Check sheet for the modelled part. Datum: model origin and axes. Units: mm. Face numbers are marked on the shaded views. Round coordinates to 2 decimals unless told otherwise and drop trailing zeros. Write each loop counter-clockwise with the first axis right and the second up, starting at its lowest first coordinate (ties: lowest second). Pieces come first, ordered by that corner, then holes. Notation, with made-up numbers: (8, 23) -> (39, 23) arc R20 cw to (39, 37) -> close; hole circle Ø2 at (-28.5, -16.5). An arc over 180 degrees is marked (long way). One line per item, written item: value.
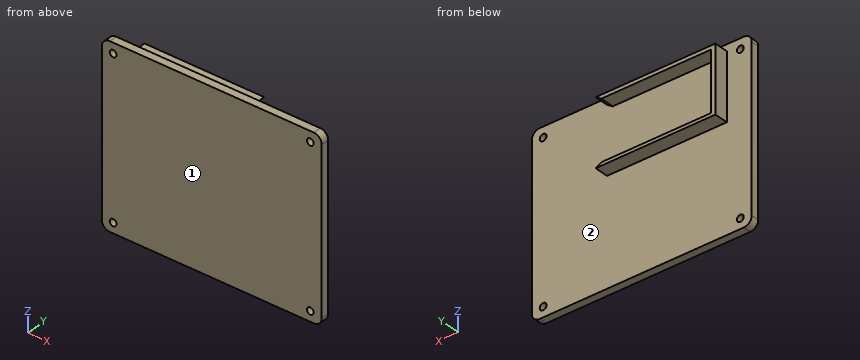
from build123d import *

# Parameters (mm, degrees)
BOSS_EXTRUDE1_DEPTH = 11
SKETCH1_3_R         = 1.7
BOSS_EXTRUDE2_DEPTH = 4


with BuildPart() as part:
    # Sketch1 → Boss-Extrude1 (new body)
    with BuildSketch(Plane(origin=(0, 0, 0), x_dir=(1, 0, 0), z_dir=(0, 1, 0))):
        Polygon((14.535232679, 29.5), (17.346594298, 31.108605337), (-42.592792902, 31.108605337), (-42.592792902, -1.87579117), (17.346594298, -1.87579117), (14.535232679, 0), (-40.464767321, 0), (-40.464767321, 29.5), align=None)
    extrude(amount=BOSS_EXTRUDE1_DEPTH)

    # Sketch1<3> → Boss-Extrude2 (add)
    with BuildSketch(Plane(origin=(0, 0, 0), x_dir=(1, 0, 0), z_dir=(0, 1, 0))):
        with BuildLine():
            Line((55.045, -1.09), (55.045, 79.51))
            ThreePointArc((55.045, 79.51), (53.873427125, 82.338427125), (51.045, 83.51))
            Line((51.045, 83.51), (-51.045, 83.51))
            ThreePointArc((-51.045, 83.51), (-53.873427125, 82.338427125), (-55.045, 79.51))
            Line((-55.045, 79.51), (-55.045, -1.09))
            ThreePointArc((-55.045, -1.09), (-53.873427125, -3.918427125), (-51.045, -5.09))
            Line((-51.045, -5.09), (51.045, -5.09))
            ThreePointArc((51.045, -5.09), (53.873427125, -3.918427125), (55.045, -1.09))
        make_face()
        with Locations((-49.365, 0)):
            Circle(SKETCH1_3_R, mode=Mode.SUBTRACT)
        Polygon((17.346594298, 31.108605337), (14.535232679, 29.5), (-40.464767321, 29.5), (-40.464767321, 0), (14.535232679, 0), (17.346594298, -1.87579117), (-42.592792902, -1.87579117), (-42.592792902, 31.108605337), align=None, mode=Mode.SUBTRACT)
        with Locations((49.365, 0)):
            Circle(SKETCH1_3_R, mode=Mode.SUBTRACT)
        with Locations((-49.365, 78.51)):
            Circle(SKETCH1_3_R, mode=Mode.SUBTRACT)
        with Locations((49.365, 78.51)):
            Circle(SKETCH1_3_R, mode=Mode.SUBTRACT)
    extrude(amount=BOSS_EXTRUDE2_DEPTH)


solid = part.part
Item 1: Sectioned sample at C-C (z = -41). Enter the section's corners in (x, y) (3 decimals).
Result set:
outline: (-55.045, 0) -> (55.045, 0) -> (55.045, 4) -> (-55.045, 4) -> close
Item 2: Depth check by flat-ended pin: pin 1 (5.5 mm diameter, centred on x = -3.5, y = 7, fed in from -Z); pin 2 (3.5 mm diameter, centred on x = -25.5, y = 8.5, fed in from +Z); pin 3 (4 mm diameter, centred on x = -49.365, z = -78.51, fed in from +Y); pin 4 (5.5 mm diameter, centred on y = 6, z = -10.5, fed in from +X) (3 decimals). Enter the tip coordinate at first touch or a pass-through.
Result set:
pin 1: z = -31.11
pin 2: z = 1.88
pin 3: y = 4
pin 4: x = 55.045
Item 3: Sectioned sample at B-B (x = -21). Enter the section's corners in (y, z).
Result set:
outline: (0, -83.51) -> (4, -83.51) -> (4, -31.11) -> (11, -31.11) -> (11, -29.5) -> (4, -29.5) -> (4, 0) -> (11, 0) -> (11, 1.88) -> (4, 1.88) -> (4, 5.09) -> (0, 5.09) -> close
Item 4: Material ranges on line 1 along X through (y, z) = (2.35, 0) (3 decimals); line 2 along Z through (x, y) = (-29, 8); line 3 along Y through (x, z) = (-19.5, -49), recorded low to high.
Result set:
line 1: -55.045 to -51.065, -47.665 to 47.665, 51.065 to 55.045
line 2: -31.11 to -29.5, 0 to 1.88
line 3: 0 to 4
Item 5: Release check for a two-part mould opening along Z. For the marked faces 1 and 2 record: pulls with the +Z half, pulls with the -Z half, needs draft (parallel to the pull), parting line crosses it, or undercut.
Result set:
face 1: needs draft
face 2: undercut
Item 6: Sectioned sample at D-D (x = 28.5). Enter the section's corners in (y, z), then the cut area to 3 significant figures.
Result set:
outline: (0, -83.51) -> (4, -83.51) -> (4, 5.09) -> (0, 5.09) -> close
area: 354 mm^2
Item 7: Sectioned sample at A-A (y = 9). Enter the section's corners in (x, z), then the cut area to 3 significant figures.
Result set:
outline: (-42.59, -31.11) -> (17.35, -31.11) -> (14.54, -29.5) -> (-40.46, -29.5) -> (-40.46, 0) -> (14.54, 0) -> (17.35, 1.88) -> (-42.59, 1.88) -> close
area: 267 mm^2
